Geometry: final body of the model. Coordinates: model frame, mm. Coordinates: 2 decimals unless noted, no trailing zeros. Write each loop counter-clockwise with the first axis right and the second up, starting at its lowest first coordinate (ties: lowest second). Pieces come first, ordered by that corner, then holes. Notation, with made-up numbers: (5, 60) - (61, 60) arc R29 ccw to (61, 91) - close; hole circle Ø10 at (18, 58). An arc over 180 degrees is marked (long way). Put each result on its own line as item: value.
```python
from build123d import *

# Parameters (mm, degrees)
F1_DEPTH = 5.08
F3_D     = 7.62
F4_R     = 5.08
F6_D     = 2.54
F8_D     = 7.62
F10_D    = 2.54
F12_D    = 2.54
F14_D    = 7.62
F16_D    = 7.62


# Not quite as in the source:
# - a feature names something its author has since deleted; it is built from what else it names


with BuildPart() as f1:
    # F0 (on Front) → F1 (new body)
    with BuildSketch(Plane.XZ):
        Polygon((27.4981856346, 177.8), (-177.8, 177.8), (-177.8, 127), (25.4, 127), (25.4, -127), (-177.8, -127), (-177.8, -177.8), (25.4, -177.8), (177.8, -177.8), (177.8, 177.8), align=None)
    extrude(amount=F1_DEPTH)

    # F3 (through all)
    with Locations(Plane.XZ.offset(5.08)):
        with Locations((-153.8637131453, 152.8165191412), (101.6, 0), (-153.1574577093, -153.8859605789), (157.1783274412, -156.3732177019), (157.1783274412, 148.4267822981)):
            Hole(F3_D / 2)

    # F4
    f4_edges = [f1.edges().sort_by_distance(p)[0] for p in [
        (177.8, -2.54, 177.8),
        (-177.8, -2.54, 177.8),
        (-177.8, -2.54, 127),
        (-177.8, -2.54, -127),
        (-177.8, -2.54, -177.8),
        (177.8, -2.54, -177.8),
    ]]
    fillet(f4_edges, radius=F4_R)

    # F6 (through all)
    with Locations(Plane.XZ.offset(5.08)):
        with Locations((93.9038, 0), (101.6, 7.6962), (109.2962, 0), (101.6, -7.6962), (-170.1568275641, -140.8739216598), (-144.7568275641, -140.8739216598), (-170.1568275641, -166.2739216598), (-144.7568275641, -166.2739216598), (157.1783274412, -148.6770177019), (151.850887514, -150.8189510301), (162.4951099118, -161.9376870028), (157.1783274412, -164.0694177019), (-170.2933631182, 171.3147368595), (-144.8933631182, 171.3147368595), (-144.8933631182, 145.9147368595), (-170.2933631182, 145.9147368595), (96.0876377272, 5.3707873365), (107.050479993, 5.433577301), (107.1167234014, -5.3663076089), (96.1674041077, -5.4514581821), (149.4821274412, -156.3732177019), (151.5333356816, -161.6044281234), (164.8745274412, -156.3732177019), (162.7891082701, -151.1053307507)):
            Hole(F6_D / 2)

    # F8 (through all)
    with Locations(Plane(origin=(0, 0, 0), x_dir=(-1, 0, 0), z_dir=(0, 1, 0))):
        with Locations((-158.2407057285, -121.0239678621)):
            Hole(F8_D / 2)

    # F10 (through all)
    with Locations(Plane.XZ.offset(5.08)):
        with Locations((165.9369057285, -121.0239678621), (164.0052020571, -115.9247447333), (163.4948166475, -126.6476510761), (158.2407057285, -128.7201678621), (152.5501607373, -126.2055884718), (150.5445057285, -121.0239678621), (153.1963041185, -115.2114377042), (158.2407057285, -113.3277678621)):
            Hole(F10_D / 2)

    # F12 (through all)
    with Locations(Plane.XZ.offset(5.08)):
        with Locations((32.0593006909, -147.3129242659), (37.4611556555, -144.6748753268), (43.3156022713, -146.8128675346), (45.0811556555, -152.2948753268), (43.8902415335, -157.5409770012), (38.2883101702, -159.6900522709), (32.5446762145, -157.8294336796), (30.2795823663, -152.5711715221)):
            Hole(F12_D / 2)

    # F14 (through all)
    with Locations(Plane.XZ.offset(5.08)):
        with Locations((37.7828851342, -151.951700449)):
            Hole(F14_D / 2)

    # F16 (through all)
    with Locations(Plane.XZ.offset(5.08)):
        with Locations((43.1287847459, 153.2645523548)):
            Hole(F16_D / 2)


solid = f1.part
```
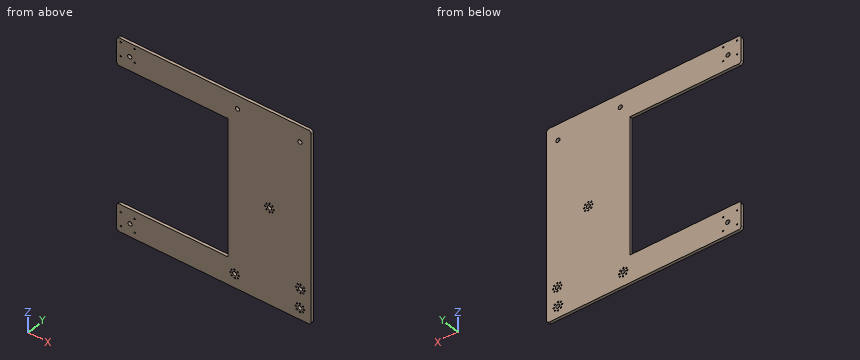
1. Section query A-A (x = 14.5). Return loops of the section in (y, z), then the cut area to 3 significant figures.
Answer below:
outline: (-5.08, -177.8) - (0, -177.8) - (0, -127) - (-5.08, -127) - close; (-5.08, 127) - (0, 127) - (0, 177.8) - (-5.08, 177.8) - close
area: 516 mm²
2. Ray query, probe 1 along Z at (x, y) = (-107, -4.25); probe 2 along Z at (x, y) = (160.5, -1.35); probe 3 along Z at (x, y) = (153, -3.9). Return the intervals inside material, ascending. Write a range as from..to.
Answer below:
probe 1: z = -177.8..-127, 127..177.8
probe 2: z = -177.8..-158.24, -154.51..-124.09, -117.96..146.56, 150.29..177.8
probe 3: z = -177.8..-151.36, -150.28..-127.39, -125.02..-116.47, -113.96..177.8
3. Section query B-B (z = 82). Return loops of the section in (x, y), then the cut area to 3 significant figures.
Answer below:
outline: (25.4, -5.08) - (177.8, -5.08) - (177.8, 0) - (25.4, 0) - close
area: 774 mm²
4. Pin query (flat end, axial travel): pin 1 Ø2 at (x, z) = (32.54, -157.83) entering from -Y; pin 2 Ø1.5 at (y, z) = (-2.5, 32) entering from -X. Return the tip coordinate at first contact, or that it passes through.
Answer below:
pin 1: passes through
pin 2: stops at x = 25.4
